```python
from build123d import *
from OCP.BRepFilletAPI import BRepFilletAPI_MakeChamfer

# Parameters (mm, degrees)
BOSS_EXTRUDE1_DEPTH      = 1.5875
BOSS_EXTRUDE1_DEPTH_BACK = 1.5875
SKETCH3_R                = 12.7
SKETCH3_R_2              = 6.3754
CHAMFER1_SIZE            = 0.254
CHAMFER1_SIZE2           = 0.439940905
CHAMFER2_SIZE            = 0.254
CHAMFER2_SIZE2           = 0.495866606


with BuildPart() as part:
    # Sketch3 → Boss-Extrude1 (new, two sides: drawn at the far end of the back side and taken through both)
    with BuildSketch(Plane.XY.offset(-BOSS_EXTRUDE1_DEPTH_BACK)):
        Circle(SKETCH3_R)
        Circle(SKETCH3_R_2, mode=Mode.SUBTRACT)
    extrude(amount=BOSS_EXTRUDE1_DEPTH + BOSS_EXTRUDE1_DEPTH_BACK)

    # Chamfer1: one chamfer whose edges measure the first distance from different faces: ONE call of the kernel's chamfer builder (chamfer() names one face for all edges)
    chamfer1_edges_1 = [part.edges().sort_by_distance(p)[0] for p in [
        (-12.7, 0, 1.5875),
    ]]
    chamfer1_side_1 = [part.faces().sort_by_distance(p)[0] for p in [
        (-12.7, 0, 0.79375),
    ]]
    chamfer1_edges_2 = [part.edges().sort_by_distance(p)[0] for p in [
        (-12.7, 0, -1.5875),
    ]]
    chamfer1_side_2 = [part.faces().sort_by_distance(p)[0] for p in [
        (-12.7, 0, -0.79375),
    ]]
    chamfer1 = BRepFilletAPI_MakeChamfer(part.part.solid().wrapped)
    for e in chamfer1_edges_1:
        chamfer1.Add(CHAMFER1_SIZE, CHAMFER1_SIZE2, e.wrapped, chamfer1_side_1[0].wrapped)  # the first distance lies on this face
    for e in chamfer1_edges_2:
        chamfer1.Add(CHAMFER1_SIZE, CHAMFER1_SIZE2, e.wrapped, chamfer1_side_2[0].wrapped)  # the first distance lies on this face
    add(Compound.cast(chamfer1.Shape()), mode=Mode.REPLACE)

    # Sketch4 → Cut-Revolve1 (revolve, cut)
    with BuildSketch(Plane(origin=(0, 0, 0), x_dir=(0, 0, -1), z_dir=(1, 0, 0)), mode=Mode.PRIVATE) as cut_revolve1_sk:
        with BuildLine():
            Line((-1.5875, 6.3246), (-1.5875, 6.4262))
            ThreePointArc((-1.5875, 6.4262), (0, 6.3754), (1.5875, 6.4262))
            Line((1.5875, 6.4262), (1.5875, 6.3246))
            Line((1.5875, 6.3246), (-1.5875, 6.3246))
        make_face()
    revolve(cut_revolve1_sk.sketch.rotate(Axis((0, 0, 1.5875), (0, 0, -1)), 90), axis=Axis((0, 0, 1.5875), (0, 0, -1)), mode=Mode.SUBTRACT)

    # Chamfer2: one chamfer whose edges measure the first distance from different faces: ONE call of the kernel's chamfer builder (chamfer() names one face for all edges)
    chamfer2_edges_1 = [part.edges().sort_by_distance(p)[0] for p in [
        (-6.4262, 0, -1.5875),
    ]]
    chamfer2_side_1 = [part.faces().sort_by_distance(p)[0] for p in [
        (-6.38810325, 0, -0.794156296),
    ]]
    chamfer2_edges_2 = [part.edges().sort_by_distance(p)[0] for p in [
        (-6.4262, 0, 1.5875),
    ]]
    chamfer2_side_2 = [part.faces().sort_by_distance(p)[0] for p in [
        (-6.38810325, 0, 0.794156296),
    ]]
    chamfer2 = BRepFilletAPI_MakeChamfer(part.part.solid().wrapped)
    for e in chamfer2_edges_1:
        chamfer2.Add(CHAMFER2_SIZE, CHAMFER2_SIZE2, e.wrapped, chamfer2_side_1[0].wrapped)  # the first distance lies on this face
    for e in chamfer2_edges_2:
        chamfer2.Add(CHAMFER2_SIZE, CHAMFER2_SIZE2, e.wrapped, chamfer2_side_2[0].wrapped)  # the first distance lies on this face
    add(Compound.cast(chamfer2.Shape()), mode=Mode.REPLACE)


solid = part.part
```
Here's how the part is built. I have some questions about the finished solid (model axes, mm). Round coordinates to 2 decimals unless told otherwise and drop trailing zeros. Write each loop counter-clockwise with the first axis right and the second up, starting at its lowest first coordinate (ties: lowest second). Pieces come first, ordered by that corner, then holes.
Q1. Please list where these lines run through material, in increasing order: probe 1 along Y at (x, z) = (1.5, 0.25); probe 2 along X at (y, z) = (2.5, -0.65); probe 3 along X at (y, z) = (3.25, -1.25).
Q2. If we section it at B-B on z = -0.8: Write out the boundary of the cut face in (x, y).
Q3. If we section it at A-A on z = 0.55: Write out the boundary of the cut face in (x, y), plus the area to 3 significant figures.
Answer below:
1. probe 1: y = -12.61 to -6.2, 6.2 to 12.61
1. probe 2: x = -12.45 to -5.87, 5.87 to 12.45
1. probe 3: x = -12.28 to -5.52, 5.52 to 12.28
2. outline: circle Ø25.4 at (0, 0); hole circle Ø12.78 at (0, 0)
3. outline: circle Ø25.4 at (0, 0); hole circle Ø12.76 at (0, 0)
3. area: 379 mm2
